Source: CAD feature listing. Evaluate the final solid. Frame: model axes, mm. A direction names the side the tool comes from. Give positions to 0.01 mm unless a question says otherwise; leave off trailing zeros. Write each loop counter-clockwise with the first axis right and the second up, starting at its lowest first coordinate (ties: lowest second). Pieces come first, ordered by that corner, then holes.
```python
from build123d import *

# Parameters (mm, degrees)
F0_W     = 6.5
F0_H     = 0.8
F1_DEPTH = 33
F2_SIZE  = 1
F3_R     = 2
F4_R     = 0.5


with BuildPart() as f1:
    # F0 (on Top) → F1 (new body)
    with BuildSketch(Plane.XY):
        with BuildLine():
            Line((-5, -24.553516), (-5, -15.5))
            Line((-5, -15.5), (-11.5, -15.5))
            Line((-11.5, -15.5), (-15, -15.5))
            Line((-15, -15.5), (-15, 15.5))
            Line((-15, 15.5), (5, 15.5))
            Line((5, 15.5), (5, 13.7))
            Line((5, 13.7), (15, 13.7))
            Line((15, 13.7), (15, 15.5))
            Line((15, 15.5), (15, 18.5))
            ThreePointArc((15, 18.5), (14.414214, 19.914214), (13, 20.5))
            Line((13, 20.5), (-20, 20.5))
            ThreePointArc((-20, 20.5), (-21.414214, 19.914214), (-22, 18.5))
            Line((-22, 18.5), (-22, -11.10081))
            ThreePointArc((-22, -11.10081), (-22.387548, -12.284026), (-23.4, -13.008688))
            ThreePointArc((-23.4, -13.008688), (-27.942683, -13.782584), (-32.526316, -13.308041))
            ThreePointArc((-32.526316, -13.308041), (-34.235442, -13.678342), (-35, -15.251137))
            Line((-35, -15.251137), (-35, -18.432774))
            Line((-35, -18.432774), (-35, -24.553516))
            ThreePointArc((-35, -24.553516), (-34.154701, -26.18651), (-32.333333, -26.439135))
            ThreePointArc((-32.333333, -26.439135), (-20, -24.323069), (-7.666667, -26.439135))
            ThreePointArc((-7.666667, -26.439135), (-5.845299, -26.18651), (-5, -24.553516))
        make_face()
        with Locations((-8.25, -15.1)):
            Rectangle(F0_W, F0_H)
    extrude(amount=F1_DEPTH)

    # F2
    f2_edges = [f1.edges().sort_by_distance(p)[0] for p in [
        (-20, -24.323069, 33),
        (-5.845299, -26.18651, 33),
        (-5, -19.626758, 33),
        (-8.25, -14.7, 33),
        (-11.5, -15.1, 33),
        (-13.25, -15.5, 33),
        (-15, 0, 33),
        (-5, 15.5, 33),
        (5, 14.6, 33),
        (10, 13.7, 33),
        (15, 16.1, 33),
        (14.414214, 19.914214, 33),
        (-3.5, 20.5, 33),
        (-21.414214, 19.914214, 33),
        (-22, 3.699595, 33),
        (-22.387548, -12.284026, 33),
        (-27.942683, -13.782584, 33),
        (-34.235442, -13.678342, 33),
        (-35, -19.902327, 33),
        (-34.154701, -26.18651, 33),
        (-20, -24.323069, 0),
        (-5.845299, -26.18651, 0),
        (-5, -19.626758, 0),
        (-8.25, -14.7, 0),
        (-11.5, -15.1, 0),
        (-13.25, -15.5, 0),
        (-15, 0, 0),
        (-5, 15.5, 0),
        (5, 14.6, 0),
        (10, 13.7, 0),
        (15, 16.1, 0),
        (14.414214, 19.914214, 0),
        (-3.5, 20.5, 0),
        (-21.414214, 19.914214, 0),
        (-22, 3.699595, 0),
        (-22.387548, -12.284026, 0),
        (-27.942683, -13.782584, 0),
        (-34.235442, -13.678342, 0),
        (-35, -19.902327, 0),
        (-34.154701, -26.18651, 0),
    ]]
    chamfer(f2_edges, length=F2_SIZE)

    # F3
    f3_edges = [f1.edges().sort_by_distance(p)[0] for p in [
        (-5, -14.7, 16.5),
        (15, 13.7, 16.5),
    ]]
    fillet(f3_edges, radius=F3_R)

    # F4
    f4_edges = [f1.edges().sort_by_distance(p)[0] for p in [
        (-11.5, -14.7, 16.5),
        (-15, -15.5, 16.5),
        (-15, 15.5, 16.5),
        (5, 13.7, 16.5),
        (5, 15.5, 16.5),
    ]]
    fillet(f4_edges, radius=F4_R)


solid = f1.part
```
1. Cut plane C-C, the plane z = 13.5. Return the cut outline in (x, y).
2. Line query: L1, parallel to Y at x = -4.5, z = 29; L2, parallel to X at y = -18, z = 5; L3, parallel to Y at x = 6, z = 15. Output: solid intervals per line, ascending.
3. Cut plane B-B, the plane x = 10. Return the cut outline in (y, z).
4. Access query for faces 4 (the flat face through (-5, -21, 16)), 5 (the flat face through (5.4, 15.2, 0.6)), 6 (the flat face through (-22, 4, 16)), 7 (the flat face through (5.4, 15.2, 32.4)), 8 (the cylindrical face through (-5.57, -15.3, 16.73)). Directions: +Z, -Z, +X, -X, +Y, -Y. A direction counts if a zero-diameter tool reaches every point of the face in a straight line with its end or side. Return the directions, or none.
5. Mould query, pull axis Y, two halves, no side actions, for faces 1 (the flat face through (-17, -5, 33)), 2 (the flat face through (-5.2, 15.9, 32.4)), 3 (the cylindrical face through (-22.4, -12.3, 16.3)). Classes: +Y half, -Y half, draft (parallel to the pull), parting line (faces both ways), or undercut.
6. Cut plane A-A, the plane y = -18.5. Return the cut outline in (x, z).
7. Contact query for flat-ended pins moving along their axis: P1, Ø2, axis at y = -5.5, z = 9, coming from the +X side; P2, Ø15, axis at y = 7.5, z = 21.5, coming from the -X side; P3, Ø12, axis at x = -29, z = 24, coming from the +Y side; P4, Ø15, axis at x = -5.5, z = 16.5, coming from the -Y side. Output: stop coordinate, or through.
Response values:
1. outline: (-35, -24.55) arc R2 ccw to (-32.33, -26.44) arc R37 cw to (-7.67, -26.44) arc R2 ccw to (-5, -24.55) - (-5, -16.7) arc R2 ccw to (-7, -14.7) - (-11, -14.7) arc R0.5 ccw to (-11.5, -15.2) - (-11.5, -15.5) - (-14.5, -15.5) arc R0.5 cw to (-15, -15) - (-15, 15) arc R0.5 cw to (-14.5, 15.5) - (4.5, 15.5) arc R0.5 cw to (5, 15) - (5, 14.2) arc R0.5 ccw to (5.5, 13.7) - (13, 13.7) arc R2 ccw to (15, 15.7) - (15, 18.5) arc R2 ccw to (13, 20.5) - (-20, 20.5) arc R2 ccw to (-22, 18.5) - (-22, -11.1) arc R2 cw to (-23.4, -13.01) arc R17 cw to (-32.53, -13.31) arc R2 ccw to (-35, -15.25) - close
2. L1: y = 15.5 to 20.5
2. L2: x = -35 to -5
2. L3: y = 13.7 to 20.5
3. outline: (13.7, 1) - (14.7, 0) - (19.5, 0) - (20.5, 1) - (20.5, 32) - (19.5, 33) - (14.7, 33) - (13.7, 32) - close
4. face 4: +Z, -Z, +X, -Y
4. face 5: -Z, -Y
4. face 6: +Z, -Z, -X, +Y
4. face 7: +Z, -Y
4. face 8: +Z, -Z, +X
5. face 1: draft
5. face 2: undercut
5. face 3: +Y half
6. outline: (-35, 1) - (-34, 0) - (-6, 0) - (-5, 1) - (-5, 32) - (-6, 33) - (-34, 33) - (-35, 32) - close
7. P1: stops at x = -15
7. P2: stops at x = -22
7. P3: stops at y = -12.83
7. P4: stops at y = -26.55
